Autodesk Inventor part; units mm, degrees
ref_plane "YZ Plane" through (0, 0, 0) normal (1, 0, 0) x (0, 1, 0)
ref_plane "XZ Plane" through (0, 0, 0) normal (0, 1, 0) x (-1, 0, 0)
ref_plane "XY Plane" through (0, 0, 0) normal (0, 0, 1) x (1, 0, 0)
ref_plane "РабПлоскость1" through (0, 0, -194) normal (0, 0, -1) x (-1, 0, 0)
sketch "Эскиз1" plane through (0, 0, -194) normal (0, 0, -1) x (-1, 0, 0)
  circle A0 centre (0, 0) radius 12
  dimension "d0" = 24
extrude "Выдавливание1" add sketch "Эскиз1" along normal blind 2
sketch "Эскиз2" plane through (0, 0, -196) normal (0, 0, -1) x (-1, 0, 0)
  circle A0 centre (0, 0) radius 14
  dimension "d3" = 28
extrude "Выдавливание2" add sketch "Эскиз2" along normal blind 2
sketch "Эскиз3" plane through (0, 0, -194) normal (0, 0, 1) x (1, 0, 0)
  line L0 (0, -14.0792) -> (7.9343, -14.0792)
  arc A0 (-0.2531, 24.5019) -> (-1.2854, 24.456) centre (0.2785, 0.9208) ccw
  line L1 (0.2785, 0.9208) -> (0.2785, 84.4485) construction
  line L2 (50, 13.9208) -> (23, 13.9208)
  line L3 (0, -14.0792) -> (50, -14.0792)
  line L4 (50, -14.0792) -> (50, 13.9208)
  line L5 (50, 13.9208) -> (0, -14.0792) construction
  line L6 (0, 13.9208) -> (50, -14.0792) construction
  line L7 (16, 53.9208) -> (-12, 53.9208)
  line L8 (16, 22.4208) -> (16, 53.9208)
  line L9 (16, 53.9208) -> (-9.7913, 3.9696) construction
  line L10 (-12, 53.9208) -> (16, -5.6793) construction
  arc A1 (16, 22.4208) -> (23, 13.9208) centre (23.4314, 21.4084) ccw
  line L11 (-7.3772, -14.0792) -> (-60, -33.2323)
  line L12 (-60, -33.2323) -> (-66.8404, -14.4385)
  line L13 (-66.8404, -14.4385) -> (-40.9989, -5.0329)
  line L14 (0, -14.0792) -> (-7.3772, -14.0792)
  arc A2 (-40.9989, -5.0329) -> (-12, 33.9208) centre (-52.4998, 33.7998) ccw
  line L15 (-12, 53.9208) -> (-12, 33.9208)
  arc A3 (1.8425, 24.456) -> (0.8102, 24.5019) centre (0.2785, 0.9208) ccw
  point P0 (0, 0)
  point P1 (0, 13.9208)
  point P2 (-24.4429, -0.0792)
  point P3 (-25, 0)
  point P4 (-0.7823, 25.5269)
  point P5 (0, 0)
  point P6 (25, -0.0792)
  point P7 (25.5571, 0)
  point P8 (1.3394, 25.5269)
  dimension "d21" = 28
  dimension "d22" = 28
  dimension "d23" = 20
  dimension "d24" = 50
  dimension "d25" = 110
  dimension "d26" = 160
  dimension "d27" = 40
  dimension "d28" = 27
  dimension "d29" = 31.5
  dimension "d30" = 20
  dimension "d31" = 27.5
  dimension "d32" = 56
  dimension "d33" = 40.5
  dimension "d34" = 7.5
  dimension "d35" = 34
  dimension "d36" = 53
  dimension "d37" = 50
extrude "Выдавливание3" add sketch "Эскиз3" along normal blind 1.8
properties part number "ЛЦМК000002.00.00.00.00.08"
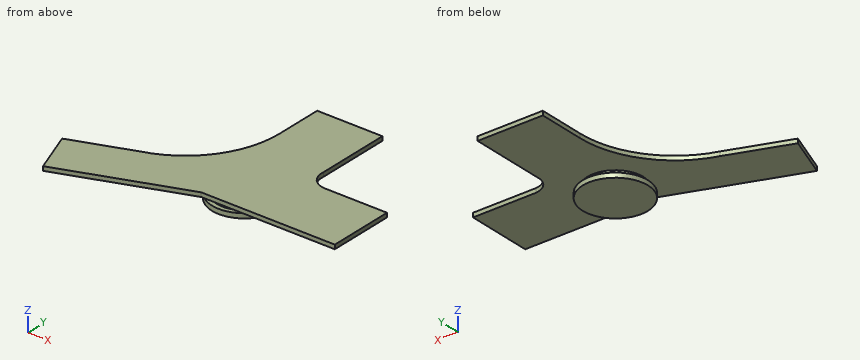
Work out the finished part from the listing and answer in its coordinate system (mm). Round coordinates to 2 decimals unless told otherwise and drop trailing zeros. Loops run counter-clockwise (first coordinate to the right, second up) from the corner with the lowest first, then second, coordinate; pieces in that order, holes last. Notation, with made-up numbers: (12.25, -12) -> (22.25, -12) arc R25 cw to (22.25, 4) -> close; hole circle Ø7 at (57.25, -12). An arc over 180 degrees is marked (long way). Write each question's results on one line, items separated by ' | '. Start each with the question number.
1. Section C-C (y = 44) is taken. Determine the outline of the cut face in (x, z).
2. Section D-D (y = -9.5) is taken. Determine the outline of the cut face in (x, z), plus the area to 3 significant figures.
3. Section A-A (x = 0) is taken. Determine the outline of the cut face in (y, z), plus the area to 3 significant figures.
4. Find the intervals of material crossed by probe 1 along Z at (x, y) = (-2.5, 31); probe 2 along Y at (x, z) = (33.5, -193.7); probe 3 along X at (y, z) = (-6.5, -196.15), in increasing order. Write a range as from..to.
5. Section B-B (z = -197) is taken. Determine the outline of the cut face in (x, y), plus the area to 3 significant figures.
6. Given pin 1 Ø2 at (x, z) = (11.5, -193.5) entering from -Y; pin 2 Ø2 at (y, z) = (36, -193.5) entering from +X; pin 3 Ø2 at (y, z) = (17.5, -194) entering from +X; pin 4 Ø1.5 at (x, z) = (20.5, -195) entering from +Y, each flat-ended and moving along its own axis, determine where each tip first touches the part or whether it passes through.
Evaluation:
1) outline: (-12, -194) -> (16, -194) -> (16, -192.2) -> (-12, -192.2) -> close
2) outline: (-53.27, -194) -> (-7.33, -194) -> (-7.33, -196) -> (-10.28, -196) -> (-10.28, -198) -> (10.28, -198) -> (10.28, -196) -> (7.33, -196) -> (7.33, -194) -> (50, -194) -> (50, -192.2) -> (-53.27, -192.2) -> close | area: 256 mm2
3) outline: (-14.08, -194) -> (-12, -194) -> (-12, -196) -> (-14, -196) -> (-14, -198) -> (14, -198) -> (14, -196) -> (12, -196) -> (12, -194) -> (53.92, -194) -> (53.92, -192.2) -> (-14.08, -192.2) -> close | area: 226 mm2
4) probe 1: z = -194..-192.2 | probe 2: y = -14.08..13.92 | probe 3: x = -12.4..12.4
5) outline: circle Ø28 at (0, 0) | area: 616 mm2
6) pin 1: stops at y = -14.08 | pin 2: stops at x = 16 | pin 3: stops at x = 17.76 | pin 4: passes through
